Read the model definition and answer for the solid it produces. Units are mm, in the model's axes. Face numbers are marked on the shaded views. A direction names the side the tool comes from. Coordinates: 2 decimals unless noted, no trailing zeros. Write each loop counter-clockwise with the first axis right and the second up, starting at its lowest first coordinate (ties: lowest second). Pieces come first, ordered by that corner, then holes.
(1) Find the intervals of material crossed by probe 1 along Y at (x, z) = (6.35, 4.75) (3 decimals); probe 2 along X at (y, z) = (19.05, 3.25) (3 decimals); probe 3 along Y at (x, z) = (38.1, 11.7) (3 decimals), in increasing order.
(2) Section C-C on y = 0 is taken. Write down the section's boundary in (x, z) (3 decimals).
(3) The mould has two halves that part along X. Classify the marked faces 3, 4, 5 and 6: +X half, -X half, draft (parallel to the pull), parting line (faces both ways), or undercut.
(4) Section A-A on z = 7 is taken. Write down the section's boundary in (x, y) (3 decimals), then the cut area to 3 significant figures.
(5) Section B-B on x = 6.35 is taken. Write down the section's boundary in (y, z) (3 decimals).
(6) Which of the six approach directions +Z, -Z, +X, -X, +Y, -Y give full straight-line access (tool end or side, diameter ignored) to the marked faces 1 and 2?
(7) Given pin 1 (2 mm diameter, centred on x = 26, y = 10.5, fed in from -Z); pin 2 (4.5 mm diameter, centred on x = 6.35, y = 19.05, fed in from +Z); pin 3 (3 mm diameter, centred on x = 36.5, y = -17, fed in from +Z); pin 4 (1.5 mm diameter, centred on x = -37, z = 19, fed in from +Y), each flat-ended and moving along its own axis, determine where each tip first touches the part or whether it passes through.
(8) Section D-D on x = 28.5 is taken. Write down the section's boundary in (y, z), then the cut area to 3 significant figures.
Autodesk Inventor part; units mm, degrees
ref_plane "YZ Plane" through (0, 0, 0) normal (1, 0, 0) x (0, 1, 0)
ref_plane "XZ Plane" through (0, 0, 0) normal (0, 1, 0) x (-1, 0, 0)
ref_plane "XY Plane" through (0, 0, 0) normal (0, 0, 1) x (1, 0, 0)
sketch "Sketch1" plane through (0, 0, 0) normal (0, 0, 1) x (1, 0, 0)
  line L0 (-273.2587, 58.9048) -> (-103.4873, 58.9048) construction
  line L1 (-103.4873, 58.9048) -> (-103.4873, -61.7557) construction
  line L2 (-103.4873, -61.7557) -> (-273.2587, -61.7557) construction
  line L3 (-273.2587, -61.7557) -> (-273.2587, 58.9048) construction
  line L4 (-44.45, 25.4) -> (44.45, 25.4)
  line L5 (44.45, 25.4) -> (44.45, -25.4)
  line L6 (44.45, -25.4) -> (-44.45, -25.4)
  line L7 (-44.45, -25.4) -> (-44.45, 25.4)
  line L8 (-44.45, 25.4) -> (44.45, -25.4) construction
  line L9 (44.45, 25.4) -> (-44.45, -25.4) construction
  circle A0 centre (38.1, 19.05) radius 2.555
  circle A1 centre (6.35, 19.05) radius 2.555
  line L10 (0, 0) -> (70.2377, 0)
  circle A2 centre (38.1, -19.05) radius 2.555
  circle A3 centre (6.35, -19.05) radius 2.555
  dimension "d5" = 88.9
  dimension "d6" = 50.8
  dimension "d7" = 5.11
  dimension "d8" = 6.35
  dimension "d9" = 6.35
  dimension "d11" = 5.11
extrude "Extrusion1" add sketch "Sketch1" along normal blind 12.7
sketch "Sketch2" plane through (0, 0, 12.7) normal (0, 0, 1) x (1, 0, 0)
  circle A0 centre (6.35, 19.05) radius 2.555
  circle A1 centre (6.35, 19.05) radius 4.765
  circle A2 centre (38.1, 19.05) radius 2.555
  circle A3 centre (38.1, 19.05) radius 4.765
  circle A4 centre (6.35, -19.05) radius 2.555
  circle A5 centre (6.35, -19.05) radius 4.765
  circle A6 centre (38.1, -19.05) radius 2.555
  circle A7 centre (38.1, -19.05) radius 4.765
  point P0 (0, 0)
  dimension "d19" = 9.53
  dimension "d20" = 9.53
  dimension "d21" = 9.53
  dimension "d22" = 9.53
extrude "Extrusion2" cut sketch "Sketch2" against normal blind 4 contours A0 | A1 | A2 | A3 | A4 | A5 | A6 | A7
sketch "Sketch3" plane through (0, 0, 12.7) normal (0, 0, 1) x (1, 0, 0)
  line L0 (-44.45, 25.4) -> (-44.45, -25.4)
  line L1 (-44.45, -19.05) -> (-25.4, -19.05)
  line L2 (-44.45, 19.05) -> (-25.4, 19.05)
  arc A0 (-25.4, -19.05) -> (-25.4, 19.05) centre (-25.4, 0) ccw
  line L3 (-44.45, -19.05) -> (-44.45, 19.05)
  point P0 (0, 0)
  dimension "d25" = 19.05
  dimension "d26" = 19.05
  dimension "d29" = 19.05
extrude "Extrusion3" add sketch "Sketch3" along normal blind 12.7
fillet "Face Fillet1" radius 4.5 1 edges at (-34.925, -19.05, 12.7)
sketch "Sketch4" plane through (0, 0, 25.4) normal (0, 0, 1) x (1, 0, 0)
  arc A0 (-25.4, -19.05) -> (-25.4, 19.05) centre (-25.4, 0) ccw
  line L0 (-44.45, 19.05) -> (-44.45, -19.05)
  line L1 (-44.45, -12.7) -> (-44.45, 12.7)
  point P0 (0, 0)
extrude "Extrusion4" [suppressed]
sketch "Sketch5" plane through (0, 0, 25.4) normal (0, 0, 1) x (1, 0, 0)
  arc A0 (-25.4, -19.05) -> (-25.4, 19.05) centre (-25.4, 0) ccw
  circle A1 centre (-25.4, 0) radius 12.7
  circle A2 centre (-25.4, 0) radius 9.525
  point P0 (0, 0)
  dimension "d38" = 25.4
  dimension "d39" = 19.05
extrude "Extrusion5" add sketch "Sketch5" along normal blind 12.7
chamfer "Chamfer1" distance 6.3 angle 26.6 3 edges at (-34.925, -19.05, 25.4) (-6.35, 0, 25.4) (-34.925, 19.05, 25.4) measured on face at (-42.3333, 0, 25.4)
sketch "Sketch6" plane through (-25.4, 0, 25.4) normal (0, 0, 1) x (1, 0, 0)
  circle A0 centre (0, 0) radius 9.525
  circle A1 centre (0, 0) radius 9.525
  point P0 (25.4, 0)
properties part number "cad@49"
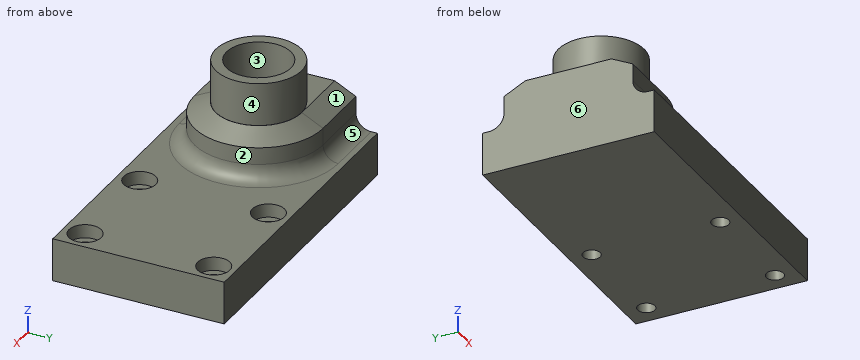
Response:
1. probe 1: y = -25.4 to -21.605, -16.495 to 16.495, 21.605 to 25.4
1. probe 2: x = -44.45 to 3.795, 8.905 to 35.545, 40.655 to 44.45
1. probe 3: y = -25.4 to -23.815, -14.285 to 14.285, 23.815 to 25.4
2. outline: (-44.45, 0) - (44.45, 0) - (44.45, 12.7) - (-1.85, 12.7) arc R4.5 cw to (-6.35, 17.2) - (-6.35, 22.245) - (-12.65, 25.4) - (-12.7, 25.4) - (-12.7, 38.1) - (-15.875, 38.1) - (-15.875, 25.4) - (-34.925, 25.4) - (-34.925, 38.1) - (-38.1, 38.1) - (-38.1, 25.4) - (-44.45, 25.4) - close
3. face 3: undercut
3. face 4: parting line
3. face 5: draft
3. face 6: -X half
4. outline: (-44.45, -25.4) - (44.45, -25.4) - (44.45, 25.4) - (-44.45, 25.4) - close; hole circle Ø5.11 at (6.35, -19.05); hole circle Ø5.11 at (6.35, 19.05); hole circle Ø5.11 at (38.1, -19.05); hole circle Ø5.11 at (38.1, 19.05)
4. area: 4,430 mm2
5. outline: (-25.4, 0) - (-21.605, 0) - (-21.605, 8.7) - (-23.815, 8.7) - (-23.815, 12.7) - (-25.4, 12.7) - close; (-16.495, 0) - (16.495, 0) - (16.495, 8.7) - (14.285, 8.7) - (14.285, 12.7) - (-14.285, 12.7) - (-14.285, 8.7) - (-16.495, 8.7) - close; (21.605, 0) - (25.4, 0) - (25.4, 12.7) - (23.815, 12.7) - (23.815, 8.7) - (21.605, 8.7) - close
6. face 1: +Z, +X, -X, +Y
6. face 2: +Z, +X
7. pin 1: stops at z = 0
7. pin 2: passes through
7. pin 3: stops at z = 8.7
7. pin 4: stops at y = 19.05
8. outline: (-25.4, 0) - (25.4, 0) - (25.4, 12.7) - (-25.4, 12.7) - close
8. area: 645 mm2
